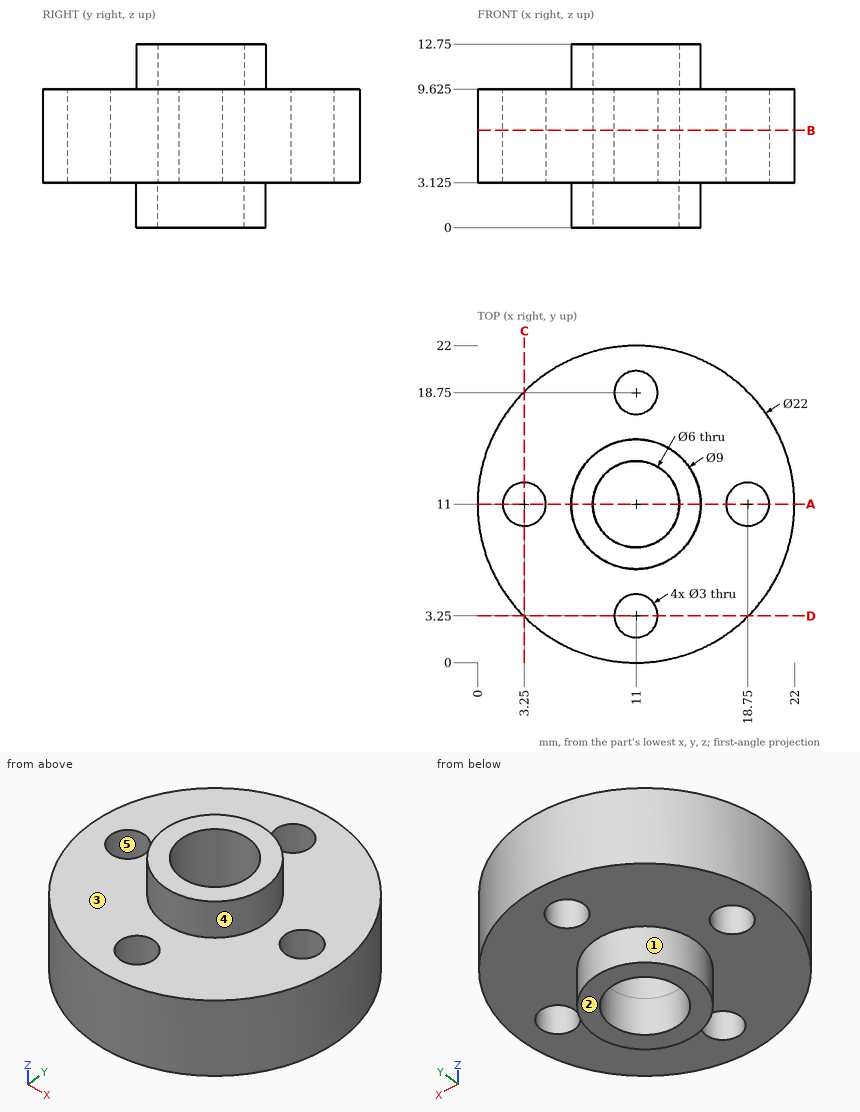
Study the drawing (mm; zero at the part's minimum x, y, z) and answer. A direction names the side the tool comes from. Give positions to 0.01 mm unless a question says otherwise; leave off trailing zeros. Loops run counter-clockwise (first coordinate to the right, second up) from the corner with the lowest first, then second, coordinate; pieces in that order, holes last. Notation, with made-up numbers: (8, 83) -> (32, 83) arc R37 cw to (32, 120) -> close; hole circle Ø6 at (44, 44.5). An arc over 180 degrees is marked (long way). Write item = value, one per line. Start each with the question number.
(1) Which of the six approach directions +Z, -Z, +X, -X, +Y, -Y give full straight-line access (tool end or side, diameter ignored) to the marked faces 1 and 2?
(2) Find the intervals of material crossed by probe 1 along Y at (x, z) = (11, 6.25); probe 2 along Y at (x, z) = (11, 1.35); probe 3 along Z at (x, y) = (9, 17.25) (3 decimals), in increasing order. Write a range as from..to.
(3) Given pin 1 Ø6 at (y, z) = (18, 2.5) entering from -X; pin 2 Ø2 at (y, z) = (8.5, 9) entering from +X, each flat-ended and moving along its own axis, determine where each tip first touches the part or whether it passes through.
(4) Find section C-C on x = 3.25. Give the vertices of the cut face in (y, z) (3 decimals).
(5) Find section A-A on y = 11. Give the vertices of the cut face in (x, z) (3 decimals), and give its area (4 significant figures).
(6) The mould has two halves that part along X. Classify the marked faces 3, 4 and 5: +X half, -X half, draft (parallel to the pull), parting line (faces both ways), or undercut.
(7) Find section B-B on z = 6.75. Give the vertices of the cut face in (x, y).
From the geometry:
q1.face_1 = -Z
q1.face_2 = -Z, +X, -X, +Y, -Y
q2.probe_1 = 0..1.75, 4.75..8, 14..17.25, 20.25..22
q2.probe_2 = 6.5..8, 14..15.5
q2.probe_3 = 3.125..9.625
q3.pin_1 = 0.78
q3.pin_2 = 21.9
q4.outline = (3.194, 3.125) -> (9.5, 3.125) -> (9.5, 9.625) -> (3.194, 9.625) -> close; (12.5, 3.125) -> (18.806, 3.125) -> (18.806, 9.625) -> (12.5, 9.625) -> close
q5.outline = (0, 3.125) -> (1.75, 3.125) -> (1.75, 9.625) -> (0, 9.625) -> close; (4.75, 3.125) -> (6.5, 3.125) -> (6.5, 0) -> (8, 0) -> (8, 12.75) -> (6.5, 12.75) -> (6.5, 9.625) -> (4.75, 9.625) -> close; (14, 0) -> (15.5, 0) -> (15.5, 3.125) -> (17.25, 3.125) -> (17.25, 9.625) -> (15.5, 9.625) -> (15.5, 12.75) -> (14, 12.75) -> close; (20.25, 3.125) -> (22, 3.125) -> (22, 9.625) -> (20.25, 9.625) -> close
q5.area = 83.75 mm^2
q6.face_3 = draft
q6.face_4 = parting line
q6.face_5 = undercut
q7.outline = circle Ø22 at (11, 11); hole circle Ø3 at (3.25, 11); hole circle Ø6 at (11, 11); hole circle Ø3 at (11, 3.25); hole circle Ø3 at (11, 18.75); hole circle Ø3 at (18.75, 11)
